from build123d import *

# Parameters (mm, degrees)
CHAMFER1_SIZE       = 1.428571429
SKETCH7_R           = 28.571428571
BOSS_EXTRUDE2_DEPTH = 4
SKETCH8_R           = 12.5
BOSS_EXTRUDE3_DEPTH = 35


with BuildPart() as part:
    # Sketch1 → Revolve1 (revolve)
    with BuildSketch(Plane.XY, mode=Mode.PRIVATE) as revolve1_sk:
        with BuildLine():
            Line((0, 0), (-30, 0))
            ThreePointArc((-30, 0), (-15.811388301, 7.434164903), (0, 10))
            Line((0, 10), (0, 0))
        make_face()
    revolve(revolve1_sk.sketch.rotate(Axis((0, 0, 0), (0, 1, 0)), 180), axis=Axis((0, 0, 0), (0, 1, 0)))

    # Chamfer1
    # the kernel refuses this chamfer: 2, 1.428571429 mm, written as the material it takes off along each edge
    with BuildSketch(Plane(origin=(0, 0, 0), x_dir=(1, 0, 0), z_dir=(0, 0, 1))) as chamfer1_piece_1:
        with BuildLine():
            Line((30 - CHAMFER1_SIZE, 0), (28.407698006, 1.14611396))
            ThreePointArc((28.407698006, 1.14611396), (29.186973853, 0.597051091), (30, 0))
            Line((30, 0), (30 - CHAMFER1_SIZE, 0))
        make_face()
    revolve(axis=Axis((0, 0, 0), (0, 1, 0)), mode=Mode.SUBTRACT)

    # Sketch7 → Boss-Extrude2 (add)
    with BuildSketch(Plane.XZ):
        with Locations(Location((0, 0, 0), (0, 0, 270))):
            Circle(SKETCH7_R)
    extrude(amount=BOSS_EXTRUDE2_DEPTH)

    # Sketch8 → Boss-Extrude3 (add)
    with BuildSketch(Plane.XZ.offset(4)):
        with Locations(Location((0, 0, 0), (0, 0, 270))):
            Circle(SKETCH8_R)
    extrude(amount=BOSS_EXTRUDE3_DEPTH)


solid = part.part
Part model, mm, in its own coordinate system. A direction names the side the tool comes from. Give positions to 0.01 mm unless a question says otherwise; leave off trailing zeros. Loops run counter-clockwise (first coordinate to the right, second up) from the corner with the lowest first, then second, coordinate; pieces in that order, holes last.
(1) Drill centre lines: line 1 along Z through (x, y) = (4, 1); line 2 along Z through (x, y) = (-2, -28.5); line 3 along Y through (x, z) = (11, 13). Where is each one in solid material? Low to high.
Return value:
line 1: z = -28.15 to 28.15
line 2: z = -12.34 to 12.34
line 3: y = -4 to 7.01
(2) 3-axis set-ups, long thin cutter, end or side, ignore diameter. For faces 1 (the flat face through (0, -39, 0)), 2 (the cylindrical face through (3.755, -21.255, -11.923)): which of +Z, -Z, +X, -X, +Y, -Y reach the whole face in a straight line?
Return value:
face 1: +Z, -Z, +X, -X, -Y
face 2: -Y
(3) Band-saw the part on A-A (x = 0). Write the cut outline in (y, z), and give its area (3 significant figures).
Return value:
outline: (-39, -12.5) - (-4, -12.5) - (-4, -28.57) - (0, -28.57) - (1.15, -28.41) arc R50 ccw to (1.15, 28.41) - (0, 28.57) - (-4, 28.57) - (-4, 12.5) - (-39, 12.5) - close
area: 1,510 mm2
(4) Band-saw the part on B-B (z = 0). Write the cut outline in (x, y), and give its area (3 significant figures).
Return value:
outline: (-28.57, -4) - (-12.5, -4) - (-12.5, -39) - (12.5, -39) - (12.5, -4) - (28.57, -4) - (28.57, 0) - (28.41, 1.15) arc R50 ccw to (-28.41, 1.15) - (-28.57, 0) - close
area: 1,510 mm2
(5) Pin check, flat tips, straight feed: pin 1 (2 mm diameter, centred on x = 18.5, z = -13, fed in from -Y); pin 2 (8 mm diameter, centred on x = -12, y = -21, fed in from -Z); pin 3 (4 mm diameter, centred on x = 7.5, y = -24, fed in from +Z) (3 decimals). Stop position of each tip, or through.
Return value:
pin 1: stops at y = -4
pin 2: stops at z = -9.6
pin 3: stops at z = 11.225
(6) Band-saw the part on C-C (y = -11). Write the cut outline in (x, z), and give its area (3 significant figures).
Return value:
outline: circle Ø25 at (0, 0)
area: 491 mm2
